```python
from build123d import *

# Parameters (mm, degrees)
SKETCH1_R               = 10
BOSS_EXTRUDE2_DEPTH     = 30
SKETCH4_R               = 10
CUT_EXTRUDE1_DEPTH      = 15
CHAMFER1_SIZE           = 20
CUT_EXTRUDE2_DEPTH      = 174.638139858
CUT_EXTRUDE2_DEPTH_BACK = 174.638139858
BOSS_EXTRUDE3_DEPTH     = 45
CUT_EXTRUDE3_DEPTH      = 198.547978004
CUT_EXTRUDE3_DEPTH_BACK = 15
SKETCH6_3_R             = 9
SKETCH8_W               = 15
SKETCH8_H               = 36
BOSS_EXTRUDE4_DEPTH     = 45.000002
SKETCH10_R              = 9
CUT_EXTRUDE4_DEPTH      = 198.547978004
BOSS_EXTRUDE5_DEPTH     = 10
CHAMFER2_SIZE           = 12
CUT_EXTRUDE5_DEPTH      = 40
CUT_EXTRUDE6_DEPTH      = 217.852953896
CUT_EXTRUDE6_DEPTH_BACK = 217.852953896
SKETCH14_OUTSIDE_W      = 287.488
SKETCH14_OUTSIDE_H      = 112.488
SKETCH14_OUTSIDE_W_2    = 100
SKETCH14_OUTSIDE_H_2    = 60
SKETCH15_R              = 10
BOSS_EXTRUDE6_DEPTH     = 10
CUT_EXTRUDE7_REACH      = 115.359


# Some blends are built 0.0001 mm under size
with BuildPart() as part:
    # Sketch1 → Boss-Extrude2 (new, symmetric)
    # profile 1 of 3: a face of its own
    with BuildSketch(Plane.XY):
        Polygon((25, -10), (-4.997737685, -45.002262315), (-25, -25), (-25, 25), (25, 25), align=None)
        Circle(SKETCH1_R, mode=Mode.SUBTRACT)
    # profile 2 of 3: a face of its own
    with BuildSketch(Plane.XY):
        Polygon((45, -10), (25, -10), (-4.997737685, -45.002262315), (45.002262315, -45.002262315), (75, -41.079226753), (75, -2.548159698), align=None)
    # profile 3 of 3: a face of its own
    with BuildSketch(Plane.XY):
        Polygon((130, 11.113547523), (75, -2.548159698), (75, -41.079226753), (130, -33.886452477), (165, -33.886452477), (165, 11.113547523), align=None)
    extrude(amount=BOSS_EXTRUDE2_DEPTH, both=True)

    # Sketch4 → Cut-Extrude1 (cut, symmetric)
    with BuildSketch(Plane.XY):
        Polygon((25, -10), (-4.997737685, -45.002262315), (-25, -25), (-25, 25), (25, 25), align=None)
        Circle(SKETCH4_R, mode=Mode.SUBTRACT)
    extrude(amount=CUT_EXTRUDE1_DEPTH, both=True, mode=Mode.SUBTRACT)

    # Chamfer1
    chamfer1_edges = [part.edges().sort_by_distance(p)[0] for p in [
        (25, -10, -22.5),
        (25, -10, 22.5),
    ]]
    chamfer(chamfer1_edges, length=CHAMFER1_SIZE - 0.0001)  # a hair under: the kernel refuses the full size

    # Sketch5 → Cut-Extrude2 (cut, two sides: drawn at the far end of the back side and taken through both)
    with BuildSketch(Plane(origin=(0, 0, 0), x_dir=(1, 0, 0), z_dir=(0, 1, 0)).offset(-CUT_EXTRUDE2_DEPTH_BACK)):
        Polygon((165, -30), (165, -18), (55.074227224, -30), align=None)
        Polygon((165, 18), (165, 30), (55.074227224, 30), align=None)
    extrude(amount=CUT_EXTRUDE2_DEPTH + CUT_EXTRUDE2_DEPTH_BACK, mode=Mode.SUBTRACT)

    # Sketch6 → Boss-Extrude3 (add)
    with BuildSketch(Plane(origin=(165, 0, 0), x_dir=(0, 0, -1), z_dir=(1, 0, 0))):
        with BuildLine():
            Line((-18, -33.886452477), (18, -33.886452477))
            Line((18, -33.886452477), (18, -17.886452477))
            ThreePointArc((18, -17.886452477), (0, -25.375680921), (-18, -17.886452477))
            Line((-18, -17.886452477), (-18, -33.886452477))
        make_face()
    extrude(amount=BOSS_EXTRUDE3_DEPTH)

    # Sketch6<3> → Cut-Extrude3 (cut, two sides: drawn at the far end of the back side and taken through both)
    with BuildSketch(Plane(origin=(165, 0, 0), x_dir=(0, 0, -1), z_dir=(1, 0, 0)).offset(-CUT_EXTRUDE3_DEPTH_BACK)):
        with Locations(Location((0, -1.886452477, 0), (0, 0, 90))):
            Circle(SKETCH6_3_R)
    extrude(amount=CUT_EXTRUDE3_DEPTH + CUT_EXTRUDE3_DEPTH_BACK, mode=Mode.SUBTRACT)

    # Sketch8 → Boss-Extrude4 (add)
    with BuildSketch(Plane.XZ.offset(33.886452477)):
        with Locations((202.5, 0)):
            Rectangle(SKETCH8_W, SKETCH8_H)
    extrude(amount=-BOSS_EXTRUDE4_DEPTH)

    # Sketch10 → Cut-Extrude4 (cut, through all)
    with BuildSketch(Plane(origin=(165, 0, 0), x_dir=(0, 0, -1), z_dir=(1, 0, 0))):
        with Locations(Location((0, -1.886452477, 0), (0, 0, 90))):
            Circle(SKETCH10_R)
    extrude(amount=CUT_EXTRUDE4_DEPTH, mode=Mode.SUBTRACT)

    # Sketch11 → Boss-Extrude5 (add)
    with BuildSketch(Plane.XZ.offset(33.886452477)):
        Polygon((130, 21.82076004), (130, -21.82076004), (165, -18), (210, -18), (210, 18), (165, 18), align=None)
    extrude(amount=BOSS_EXTRUDE5_DEPTH)

    # Chamfer2
    # the kernel refuses this chamfer: 12 mm, written as the material it takes off along each edge
    with BuildSketch(Plane(origin=(130, -43.886452477, 52.680955896), x_dir=(-0.02749587661058907, 0.9996219169112965, 0), z_dir=(0, 0, -1))) as chamfer2_piece_1_section:
        Polygon((CHAMFER2_SIZE * 0.999621916911, CHAMFER2_SIZE * 0.0274958766106), (-CHAMFER2_SIZE * 0.0274958766106, CHAMFER2_SIZE * 0.999621916911), (0, 0), align=None)
    chamfer2_piece_1 = extrude(amount=105.361911791, mode=Mode.PRIVATE)
    chamfer2_piece_1 = split(chamfer2_piece_1, bisect_by=Plane(origin=(133.216907805, -33.465752628, 0), z_dir=(0.1296735244167249, -0.9915567442488328, 0)), keep=Keep.TOP, mode=Mode.PRIVATE)
    add(chamfer2_piece_1, mode=Mode.SUBTRACT)

    # Sketch13 → Cut-Extrude5 (cut)
    with BuildSketch(Plane.XY.offset(18)):
        with BuildLine():
            Line((165, -17.886452477), (195, -17.886452477))
            ThreePointArc((195, -17.886452477), (180, -25.224548687), (165, -17.886452477))
        make_face()
    extrude(amount=-CUT_EXTRUDE5_DEPTH, mode=Mode.SUBTRACT)

    # Sketch14 outside → Cut-Extrude6 (cut, two sides: drawn at the far end of the back side and taken through both)
    with BuildSketch(Plane(origin=(0, 0, 0), x_dir=(1, 0, 0), z_dir=(0, 1, 0)).offset(-CUT_EXTRUDE6_DEPTH_BACK)):
        with Locations((92.5, 0)):
            Rectangle(SKETCH14_OUTSIDE_W, SKETCH14_OUTSIDE_H)
        with Locations((25, 0)):
            Rectangle(SKETCH14_OUTSIDE_W_2, SKETCH14_OUTSIDE_H_2, mode=Mode.SUBTRACT)
    extrude(amount=CUT_EXTRUDE6_DEPTH + CUT_EXTRUDE6_DEPTH_BACK, mode=Mode.SUBTRACT)

    # Sketch15 → Boss-Extrude6 (add)
    with BuildSketch(Plane(origin=(75, 0, 0), x_dir=(0, 0, -1), z_dir=(1, 0, 0))):
        with Locations((0, -22.3255367)):
            Circle(SKETCH15_R)
    extrude(amount=BOSS_EXTRUDE6_DEPTH)

    # Cut-Extrude7: up to this face of the body (flat: up to its plane)
    cut_extrude7_end = Plane(part.part.faces().sort_by_distance((12.358249011, -13.375403826, 30))[0])
    # Sketch16 → Cut-Extrude7 (cut, up to the picked face)
    with BuildSketch(Plane(origin=(0, 0, -30), x_dir=(-1, 0, 0), z_dir=(0, 0, -1)), mode=Mode.PRIVATE) as cut_extrude7_sk1:
        with BuildLine():
            Line((-8.033000326, 25), (-4.250478251, 9.051708935))
            ThreePointArc((-4.250478251, 9.051708935), (0.734596104, 9.972981929), (5.530881389, 8.331227464))
            Line((5.530881389, 8.331227464), (9.650814715, 25))
            Line((9.650814715, 25), (-8.033000326, 25))
        make_face()
    cut_extrude7_tool1 = split(extrude(cut_extrude7_sk1.sketch, amount=-CUT_EXTRUDE7_REACH, mode=Mode.PRIVATE), bisect_by=cut_extrude7_end, keep=Keep.BOTH, mode=Mode.PRIVATE)
    add(cut_extrude7_tool1.solids().sort_by(Axis((-0.802445, 17.957811, -30), (0, 0, 1)))[0], mode=Mode.SUBTRACT)


solid = part.part
```
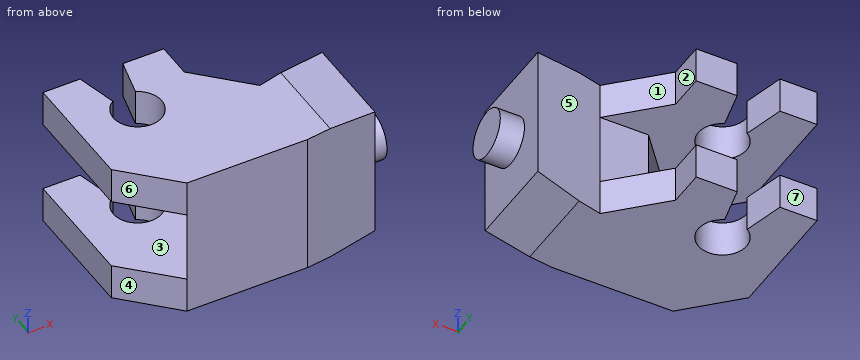
Here's how the part is built. I have some questions about the finished solid (model axes, mm). Face numbers are marked on the shaded views. A direction names the side the tool comes from. Coordinates: 2 decimals unless noted, no trailing zeros. Loops run counter-clockwise (first coordinate to the right, second up) from the corner with the lowest first, then second, coordinate; pieces in that order, holes last. Notation, with made-up numbers: (77, 51.25) - (135, 51.25) arc R36 ccw to (135, 86.25) - close; hole circle Ø2 at (33, 70). An arc over 180 degrees is marked (long way). Return JSON: item names as keys, results as strings. Group by question number.
Item 1: We'd pull the mould along X, two halves only. Please class the marked faces 5, 6 and 7: +X half, -X half, draft (parallel to the pull), parting line (faces both ways), or undercut.
Item 2: If we section it at D-D on x = 5.5: Write out the boundary of the cut face in (y, z), and give its area (3 significant figures).
Item 3: If we section it at C-C on y = 17: Write out the boundary of the cut face in (x, z), and give its area (3 significant figures).
Item 4: I need wall thicknesses on line 1 (Z direction, x = -15, y = -17.5); line 2 (Y direction, x = 0, z = 25); line 3 (X direction, y = 0, z = -26.5). Which ranges of each line are inside material? Lowest first, please. Write a range as from..to.
Item 5: On a 3-axis mill with a long thin cutter (end or side, diameter ignored), from which of +Z, -Z, +X, -X, +Y, -Y can I reach the whole of each face in a straight line? I mean the marked faces 1, 2, 3 and 4. Say none if no direction works.
Item 6: Will these pins go through, and if not, where does the flat tip stop? P1, Ø8, axis at y = -29, z = -23, coming from the +X side; P2, Ø16.5, axis at y = 17.5, z = -22, coming from the +X side; P3, Ø12, axis at x = 72, y = -38, coming from the +Z side.
Item 7: If we section it at B-B on x = -7.5: Write out the boundary of the cut face in (y, z).
Calculated:
{
 "1": {"face 5": "undercut", "face 6": "-X half", "face 7": "draft"},
 "2": {"outline": "(-45, -30) - (-8.35, -30) - (-8.35, -15) - (-32.75, -15) - (-32.75, 15) - (-8.35, 15) - (-8.35, 30) - (-45, 30) - close; (8.35, -30) - (14.32, -30) - (14.32, -15) - (8.35, -15) - close; (8.35, 15) - (14.32, 15) - (14.32, 30) - (8.35, 30) - close", "area": "1,650 mm^2"},
 "3": {"outline": "(-25, -30) - (-7.67, -30) - (-7.67, -15) - (-25, -15) - close; (-25, 15) - (-7.67, 15) - (-7.67, 30) - (-25, 30) - close; (6.14, -30) - (25, -30) - (25, -15) - (6.14, -15) - close; (6.14, 15) - (25, 15) - (25, 30) - (6.14, 30) - close", "area": "1,090 mm^2"},
 "4": {"line 1": "z = -30..-15, 15..30", "line 2": "y = -45..-10", "line 3": "x = -25..-10, 10..35"},
 "5": {"face 1": "+Z, -Z, +Y", "face 2": "+Z, -Z, +X, +Y", "face 3": "-X, +Y", "face 4": "+Z, -Z, -X, -Y"},
 "6": {"P1": "stops at x = 75", "P2": "stops at x = 25.75", "P3": "stops at z = 28.81"},
 "7": {"outline": "(-42.5, -30) - (-6.61, -30) - (-6.61, -15) - (-42.5, -15) - close; (-42.5, 15) - (-6.61, 15) - (-6.61, 30) - (-42.5, 30) - close; (6.61, -30) - (16.3, -30) - (16.3, -15) - (6.61, -15) - close; (6.61, 15) - (16.3, 15) - (16.3, 30) - (6.61, 30) - close"}
}
